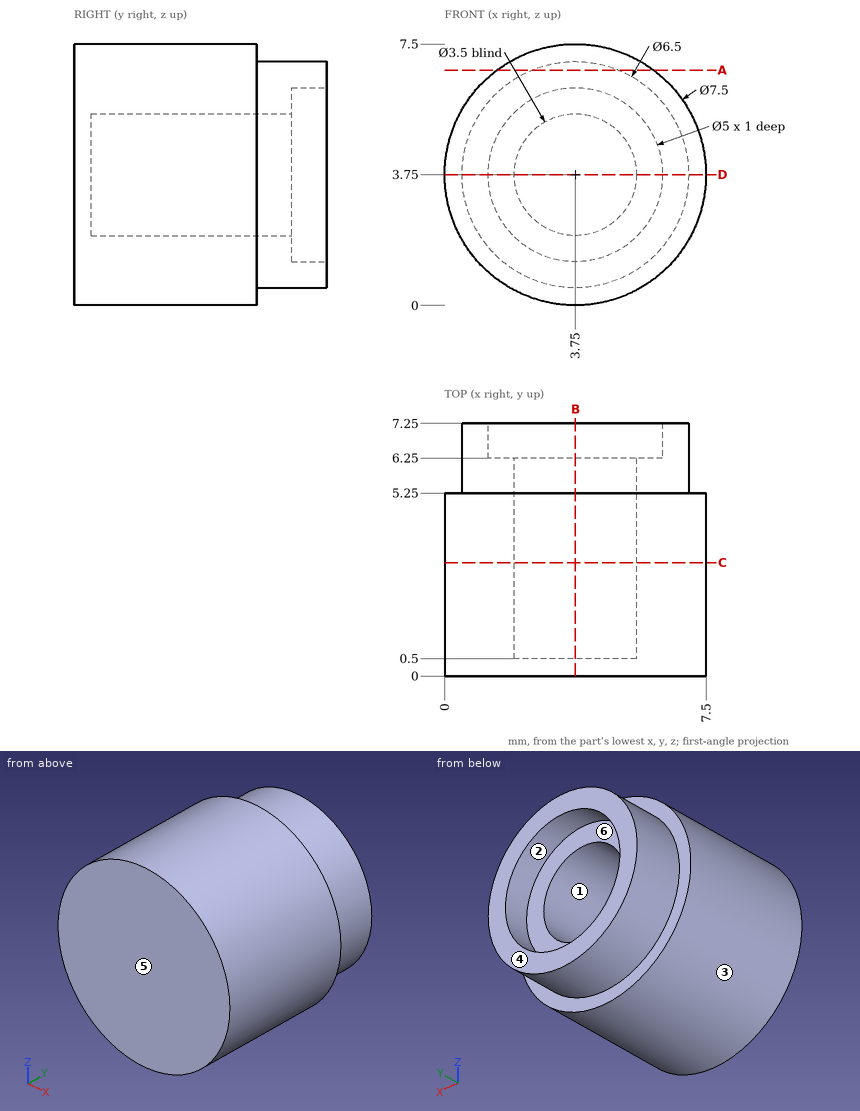
Geometry: see drawing. Coordinates: mm, zero at the bounding-box minimum. A direction names the side the tool comes from. Coordinates: 2 decimals unless noted, no trailing zeros. Order: outer loops, then holes, each group sorted by start corner. A loop starts at its lowest first (then second) coordinate and runs counter-clockwise, first axis right, second up. Notation, with made-up numbers: M 82.25,19.5 L 128.25,19.5 A34 cw 128.25,51.5 Z; hole C 28.25,-20 d2. An arc over 180 degrees is marked long. Write each question's results on one line, items separated by ' | '. Start each with the question number.
1) Access query for the marked faces 5 and 6. Directions: +Z, -Z, +X, -X, +Y, -Y. A direction counts if a zero-diameter tool reaches every point of the face in a straight line with its end or side. Return the directions, or none.
2) Contact query for flat-ended pins moving along their axis: pin 1 Ø2 at (x, z) = (2, 5) entering from +Y; pin 2 Ø1.5 at (x, z) = (4.5, 5) entering from +Y; pin 3 Ø2 at (x, z) = (3.75, 3.75) entering from +Y. Output: stop coordinate, or through.
3) Section query D-D (z = 3.75). Return the cut outline in (x, y).
4) Line query: line 1 (X direction, y = 6.65, z = 3.75); line 2 (X direction, y = 2.3, z = 3.75). Output: solid intervals per line, ascending. Write a range as from..to.
5) Section query A-A (z = 6.75). Return the cut outline in (x, y).
6) Section query B-B (x = 3.75). Return the cut outline in (y, z), plus the area to 4 significant figures.
7) Draft query along X for the marked faces 1, 2, 3 and 4. Return one class per face: released by +X, released by -X, zero draft, split by the parting line, or undercut.
8) Section query C-C (y = 3.25). Return the cut outline in (x, z), plus the area to 3 significant figures.
Answers:
1) face 5: +Z, -Z, +X, -X, -Y | face 6: +Y
2) pin 1: stops at y = 7.25 | pin 2: stops at y = 6.25 | pin 3: stops at y = 0.5
3) outline: M 0,0 L 7.5,0 L 7.5,5.25 L 7,5.25 L 7,7.25 L 6.25,7.25 L 6.25,6.25 L 5.5,6.25 L 5.5,0.5 L 2,0.5 L 2,6.25 L 1.25,6.25 L 1.25,7.25 L 0.5,7.25 L 0.5,5.25 L 0,5.25 Z
4) line 1: x = 0.5..1.25, 6.25..7 | line 2: x = 0..2, 5.5..7.5
5) outline: M 1.5,0 L 6,0 L 6,5.25 L 5,5.25 L 5,7.25 L 2.5,7.25 L 2.5,5.25 L 1.5,5.25 Z
6) outline: M 0,0 L 5.25,0 L 5.25,0.5 L 7.25,0.5 L 7.25,1.25 L 6.25,1.25 L 6.25,2 L 0.5,2 L 0.5,5.5 L 6.25,5.5 L 6.25,6.25 L 7.25,6.25 L 7.25,7 L 5.25,7 L 5.25,7.5 L 0,7.5 Z | area: 27.25 mm^2
7) face 1: undercut | face 2: undercut | face 3: split by the parting line | face 4: zero draft
8) outline: C 3.75,3.75 d7.5; hole C 3.75,3.75 d3.5 | area: 34.6 mm^2
